```python
from build123d import *

# Parameters (mm, degrees)
IZIM1_R                     = 20
Y_KSEKLIK_EKSTR_ZYON1_DEPTH = 10
IZIM2_R                     = 15
Y_KSEKLIK_EKSTR_ZYON2_DEPTH = 5
IZIM3_R                     = 20
Y_KSEKLIK_EKSTR_ZYON3_DEPTH = 15
IZIM4_R                     = 20
Y_KSEKLIK_EKSTR_ZYON4_DEPTH = 5
IZIM5_R                     = 10
KES_EKSTR_ZYON1_DEPTH       = 11
KES_EKSTR_ZYON1_DEPTH_BACK  = 21
Y_KSEKLIK_EKSTR_ZYON5_DEPTH = 5
KES_EKSTR_ZYON3_START       = -5
IZIM8_W                     = 10
IZIM8_H                     = 55.466945175
KES_EKSTR_ZYON3_DEPTH       = 90
IZIM9_R                     = 10
KES_EKSTR_ZYON4_DEPTH       = 21


with BuildPart() as part:
    # Çizim1 → Yükseklik-Ekstrüzyon1 (new body)
    with BuildSketch(Plane(origin=(0, 0, 0), x_dir=(0, 0, -1), z_dir=(1, 0, 0))):
        with BuildLine():
            Line((22.00493217, 15.116319136), (14.949905951, 101.224872265))
            ThreePointArc((14.949905951, 101.224872265), (-0.237952402, 114.998112503), (-14.981238267, 100.75))
            Line((-14.981238267, 100.75), (-19.974984355, 1))
            ThreePointArc((-19.974984355, 1), (0.500156421, 19.993745111), (20, 0))
            ThreePointArc((20, 0), (8.265673223, -18.212046732), (-13.167864617, -15.053482701))
            Line((-13.167864617, -15.053482701), (43.157110126, -64.323120614))
            ThreePointArc((43.157110126, -64.323120614), (64.073343656, -63.187367339), (63.459512577, -42.249316522))
            Line((63.459512577, -42.249316522), (37.082938713, -16.746413538))
            ThreePointArc((37.082938713, -16.746413538), (26.642905037, -2.187865906), (22.00493217, 15.116319136))
        make_face()
        Circle(IZIM1_R)
    extrude(amount=Y_KSEKLIK_EKSTR_ZYON1_DEPTH)

    # Çizim2 → Yükseklik-Ekstrüzyon2 (add)
    with BuildSketch(Plane(origin=(10, 0, 0), x_dir=(0, 0, -1), z_dir=(1, 0, 0))):
        with Locations((0, 100)):
            Circle(IZIM2_R)
    y_kseklik_ekstr_zyon2 = extrude(amount=Y_KSEKLIK_EKSTR_ZYON2_DEPTH)

    # Aynalama1: Yükseklik-Ekstrüzyon2 across plane
    add(y_kseklik_ekstr_zyon2.mirror(Plane(origin=(5, 0, 0), x_dir=(0, 0, 1), z_dir=(1, 0, 0))))

    # Çizim3 → Yükseklik-Ekstrüzyon3 (add)
    with BuildSketch(Plane(origin=(10, 0, 0), x_dir=(0, 0, -1), z_dir=(1, 0, 0))):
        Circle(IZIM3_R)
    extrude(amount=Y_KSEKLIK_EKSTR_ZYON3_DEPTH)

    # Çizim4 → Yükseklik-Ekstrüzyon4 (add)
    with BuildSketch(Plane.ZY):
        Circle(IZIM4_R)
    extrude(amount=Y_KSEKLIK_EKSTR_ZYON4_DEPTH)

    # Çizim5 → Kes-Ekstrüzyon1 (cut, two sides)
    with BuildSketch(Plane(origin=(15, 0, 0), x_dir=(0, 0, -1), z_dir=(1, 0, 0))) as kes_ekstr_zyon1_sk:
        with Locations((0, 100)):
            Circle(IZIM5_R)
        Circle(IZIM5_R)
    extrude(amount=KES_EKSTR_ZYON1_DEPTH, mode=Mode.SUBTRACT)
    extrude(kes_ekstr_zyon1_sk.sketch, amount=-KES_EKSTR_ZYON1_DEPTH_BACK, mode=Mode.SUBTRACT)

    # Çizim6 → Yükseklik-Ekstrüzyon5 (add)
    with BuildSketch(Plane(origin=(10, 0, 0), x_dir=(0, 0, -1), z_dir=(1, 0, 0))):
        with BuildLine():
            ThreePointArc((37.082938713, -16.746413538), (35.998094477, -15.664861033), (34.94689158, -14.550583103))
            Line((34.94689158, -14.550583103), (12.228664173, -37.26881051))
            Line((12.228664173, -37.26881051), (43.157110126, -64.323120614))
            ThreePointArc((43.157110126, -64.323120614), (64.073343656, -63.187367339), (63.459512577, -42.249316522))
            Line((63.459512577, -42.249316522), (37.082938713, -16.746413538))
        make_face()
    y_kseklik_ekstr_zyon5 = extrude(amount=Y_KSEKLIK_EKSTR_ZYON5_DEPTH)

    # Aynalama2: Yükseklik-Ekstrüzyon5 across plane
    add(y_kseklik_ekstr_zyon5.mirror(Plane(origin=(5, 0, 0), x_dir=(0, 0, 1), z_dir=(1, 0, 0))))

    # Çizim8 → Kes-Ekstrüzyon3 (cut)
    with BuildSketch(Plane(origin=(0, -24.748737342, -24.748737342), x_dir=(1, 0, 0), z_dir=(0, 0.707106781, 0.707106781)).offset(KES_EKSTR_ZYON3_START)):
        with Locations((5, -5.759989705)):
            Rectangle(IZIM8_W, IZIM8_H)
    extrude(amount=-KES_EKSTR_ZYON3_DEPTH, mode=Mode.SUBTRACT)

    # Çizim9 → Kes-Ekstrüzyon4 (cut, through all)
    with BuildSketch(Plane(origin=(15, 0, 0), x_dir=(0, 0, -1), z_dir=(1, 0, 0))):
        with Locations((53.033008589, -53.033008589)):
            Circle(IZIM9_R)
    extrude(amount=-KES_EKSTR_ZYON4_DEPTH, mode=Mode.SUBTRACT)


solid = part.part
```
The listing builds one solid part. Answer for the finished solid, in the listing's coordinates (mm). A direction names the side the tool comes from. Give positions to 0.01 mm unless a question says otherwise; leave off trailing zeros. Order: outer loops, then holes, each group sorted by start corner. A loop starts at its lowest first (then second) coordinate and runs counter-clockwise, first axis right, second up. Notation, with made-up numbers: (-4.75, 35) -> (54.25, 35) arc R11 ccw to (54.25, 56) -> close; hole circle Ø8 at (-22.5, 88.25). An arc over 180 degrees is marked (long way). Answer as CSV lines item,"result". Start each with the question number.
Q1. A cutting plane is placed at A-A (z = -52.5). Determine the outline of the cut face in (x, y), then the cut area to 3 significant figures.
Q2. Given pin 1 (4 mm diameter, centred on x = 7.5, y = 90.5, fed in from +Z); pin 2 (2 mm diameter, centred on x = 17.5, y = -31.5, fed in from -Z); pin 3 (3 mm diameter, centred on x = 1, y = -20.5, fed in from -Z); pin 4 (15 mm diameter, centred on y = 95, z = 3.5, fed in from +X), each flat-ended and moving along its own axis, determine where each tip first touches the part or whether it passes through.
Q3. A cutting plane is placed at D-D (y = 58). Determine the outline of the cut face in (x, z).
Q4. A cutting plane is placed at B-B (z = 0). Determine the outline of the cut face in (x, y), then the cut area to 3 significant figures.
Q5. Which of the six approach directions +Z, -Z, +X, -X, +Y, -Y give full straight-line access (tool end or side, diameter ignored) to faces 1 (the cylindrical face through (-2.465, -62.795, -50.865)), 2 (the flat face through (0, -43, -41)), 3 (the flat face through (-5, -41, -40)), 4 (the flat face through (-2.5, -25.8, -23.7)), 5 (the flat face through (15, 97, -10))?
Q6. Determine the mould class of faces 6 (the flat face through (12.5, -25.8, -23.7)), 7 (the flat face through (25, 9, 5)), 8 (the flat face through (0, 33, -1)), 9 (the flat face through (4.93, -29.17, -27.4)) for opening direction Y: pulls with the +Y half, pulls with the -Y half, needs draft (parallel to the pull), parting line crosses it, or undercut.
Q7. Find the intervals of material crossed by L1, parallel to Y at x = 0.5, z = 6.5; L2, parallel to Y at x = 8.5, z = 0; L3, parallel to X at y = -55, z = -36.5, in increasing order.
Q8. A cutting plane is placed at C-C (x = 22.5). Determine the outline of the cut face in (y, z).
Results found:
1,outline,"(-5, -68.02) -> (0, -68.02) -> (0, -63.02) -> (-5, -63.02) -> close; (-5, -43.05) -> (0, -43.05) -> (0, -31.65) -> (-5, -31.65) -> close; (10, -68.02) -> (15, -68.02) -> (15, -63.02) -> (10, -63.02) -> close; (10, -43.05) -> (15, -43.05) -> (15, -31.65) -> (10, -31.65) -> close"
1,area,"164 mm2"
2,pin 1,"z = 15.59"
2,pin 2,"through"
2,pin 3,"z = -42.12"
2,pin 4,"x = 15"
3,outline,"(0, -18.49) -> (10, -18.49) -> (10, 17.12) -> (0, 17.12) -> close"
4,outline,"(-5, -20) -> (0, -20) -> (0, -26.57) -> (10, -26.57) -> (10, -20) -> (25, -20) -> (25, -10) -> (-5, -10) -> close; (-5, 10) -> (25, 10) -> (25, 20) -> (10, 20) -> (10, 85) -> (15, 85) -> (15, 90) -> (-5, 90) -> (-5, 85) -> (0, 85) -> (0, 20) -> (-5, 20) -> close; (-5, 110) -> (15, 110) -> (15, 115) -> (-5, 115) -> close"
4,area,"1,520 mm2"
5,face 1,"+X, -X"
5,face 2,"-Z, -Y"
5,face 3,"+Z, -Z, -X, +Y, -Y"
5,face 4,"-X"
5,face 5,"+Z, -Z, +X, +Y"
6,face 6,"undercut"
6,face 7,"needs draft"
6,face 8,"undercut"
6,face 9,"pulls with the -Y half"
7,L1,"-20.89 to -7.6, 7.6 to 92.4, 107.6 to 113.52"
7,L2,"-26.57 to -10, 10 to 90, 110 to 115"
7,L3,"-5 to 0, 10 to 15"
8,outline,"circle Ø40 at (0, 0); hole circle Ø20 at (0, 0)"
